from build123d import *

# Parameters (mm, degrees)
F1_DEPTH = 4.99999
F2_R     = 2.54
F3_DEPTH = 12.7


# Not quite as in the source:
# - the program builds the solid bodies; features that only make, move or delete a surface that nothing else refers to are left out


with BuildPart() as f1:
    # F0 (on Top) → F1 (new body)
    with BuildSketch(Plane.XY):
        with BuildLine():
            Line((24.9985645242, 15.2049488522), (-27.3015594758, 15.2049488522))
            ThreePointArc((-27.3015594758, 15.2049488522), (-31.7916875363, 13.3450769127), (-33.6515594758, 8.8549488522))
            Line((-33.6515594758, 8.8549488522), (-33.6515594758, -8.4449911478))
            ThreePointArc((-33.6515594758, -8.4449911478), (-31.7916875363, -12.9351192083), (-27.3015594758, -14.7949911478))
            Line((-27.3015594758, -14.7949911478), (24.9985645242, -14.7949911478))
            ThreePointArc((24.9985645242, -14.7949911478), (29.4886925847, -12.9351192083), (31.3485645242, -8.4449911478))
            Line((31.3485645242, -8.4449911478), (31.3485645242, 8.8549488522))
            ThreePointArc((31.3485645242, 8.8549488522), (29.4886925847, 13.3450769127), (24.9985645242, 15.2049488522))
        make_face()
    extrude(amount=F1_DEPTH)

    # F2 (on Top) → F3 (cut, symmetric)
    with BuildSketch(Plane.XY):
        with Locations((-28.451833874, 10.8810858801)):
            Circle(F2_R)
        with Locations((-28.451833874, -10.7532069087)):
            Circle(F2_R)
        with Locations((26.2153949589, -10.7532069087)):
            Circle(F2_R)
        with Locations((26.2153949589, 10.8810858801)):
            Circle(F2_R)
    extrude(amount=F3_DEPTH, both=True, mode=Mode.SUBTRACT)


solid = f1.part
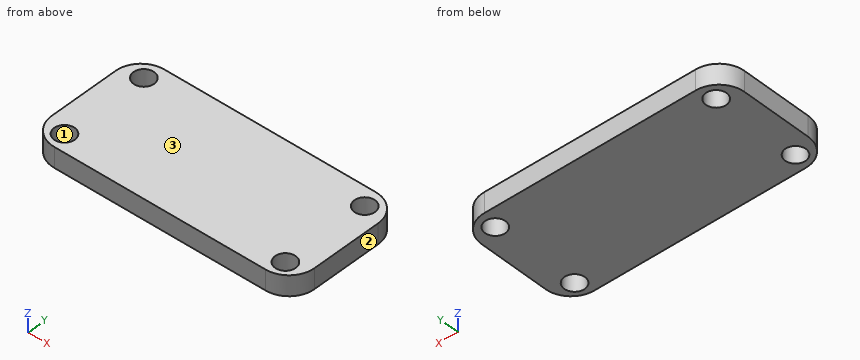
Verification items for the finished model (mm, model axes). Face numbers are marked on the shaded views. Coordinates: 2 decimals unless noted, no trailing zeros. Loops run counter-clockwise (first coordinate to the right, second up) from the corner with the lowest first, then second, coordinate; pieces in that order, holes last. Notation, with made-up numbers: (75.25, 3) -> (88.25, 3) arc R32 ccw to (88.25, 34) -> close; hole circle Ø1 at (70.5, 67). An arc over 180 degrees is marked (long way). Answer as a JSON object with one key per item and string values. Group by question number.
Item 1: Mould release check, pull along X, two halves, no side actions. Record for the marked faces 1, 2 and 3: +X half, -X half, draft (parallel to the pull), parting line (faces both ways), or undercut.
Item 2: Sectioned sample at B-B on z = 3.3. Record the boundary of the cut face in (x, y) (3 decimals), plus the area to 3 significant figures.
Item 3: Sectioned sample at A-A on y = -11.5. Record the boundary of the cut face in (x, z), plus the area to 3 significant figures.
Item 4: Scan lines: probe 1 along Y at (x, z) = (-26.5, 3.5) (1 decimal); probe 2 along Y at (x, z) = (25.5, 0.3); probe 3 along X at (y, z) = (-11.25, 2). Record each from-to range of solid material in increasing order.
Item 5: Depth check by flat-ended pin: pin 1 (6 mm diameter, centred on x = -23.5, y = -10, fed in from -Z); pin 2 (2 mm diameter, centred on y = -11.5, z = 4, fed in from -X). Enter the tip coordinate at first touch or a pass-through.
Item 6: Sectioned sample at C-C on y = 11.5. Record the boundary of the cut face in (x, z), plus the area to 3 significant figures.
Evaluation:
{
 "1": {"face 1": "undercut", "face 2": "+X half", "face 3": "draft"},
 "2": {"outline": "(-33.652, -8.445) arc R6.35 ccw to (-27.302, -14.795) -> (24.999, -14.795) arc R6.35 ccw to (31.349, -8.445) -> (31.349, 8.855) arc R6.35 ccw to (24.999, 15.205) -> (-27.302, 15.205) arc R6.35 ccw to (-33.652, 8.855) -> close; hole circle Ø5.08 at (-28.452, -10.753); hole circle Ø5.08 at (-28.452, 10.881); hole circle Ø5.08 at (26.215, -10.753); hole circle Ø5.08 at (26.215, 10.881)", "area": "1,830 mm²"},
 "3": {"outline": "(-32.87, 0) -> (-30.88, 0) -> (-30.88, 5) -> (-32.87, 5) -> close; (-26.02, 0) -> (23.79, 0) -> (23.79, 5) -> (-26.02, 5) -> close; (28.64, 0) -> (30.57, 0) -> (30.57, 5) -> (28.64, 5) -> close", "area": "269 mm²"},
 "4": {"probe 1": "y = -14.8 to -12.4, -9.1 to 9.3, 12.5 to 15.2", "probe 2": "y = -14.78 to -13.19, -8.32 to 8.44, 13.32 to 15.19", "probe 3": "x = -33 to -30.94, -25.96 to 23.72, 28.71 to 30.7"},
 "5": {"pin 1": "stops at z = 0", "pin 2": "stops at x = -33.31"},
 "6": {"outline": "(-33.07, 0) -> (-30.92, 0) -> (-30.92, 5) -> (-33.07, 5) -> close; (-25.99, 0) -> (23.75, 0) -> (23.75, 5) -> (-25.99, 5) -> close; (28.68, 0) -> (30.77, 0) -> (30.77, 5) -> (28.68, 5) -> close", "area": "270 mm²"}
}
